Design review of the part built by this model. Coordinates are the model's own, in mm. A direction names the side the tool comes from. Coordinates: 2 decimals unless noted, no trailing zeros. Order: outer loops, then holes, each group sorted by start corner. A loop starts at its lowest first (then second) coordinate and runs counter-clockwise, first axis right, second up. Notation, with made-up numbers: M 89.5,-22.75 L 122.5,-22.75 A18 ccw 122.5,7.25 Z; hole C 66.25,28 d10. An arc over 180 degrees is marked long. Answer as a JSON object with one key per item and string values.
from build123d import *

# Parameters (mm, degrees)
SKETCH1_W           = 60
SKETCH1_H           = 38
BOSS_EXTRUDE1_DEPTH = 35
SKETCH2_R           = 2.9
SKETCH2_R_2         = 3.05
CUT_EXTRUDE1_DEPTH  = 36
SKETCH3_R           = 5.5
CUT_EXTRUDE2_DEPTH  = 7
CHAMFER1_SIZE       = 0.4


with BuildPart() as part:
    # Sketch1 → Boss-Extrude1 (new body)
    with BuildSketch(Plane(origin=(0, 0, 0), x_dir=(1, 0, 0), z_dir=(0, 1, 0))):
        Rectangle(SKETCH1_W, SKETCH1_H)
    extrude(amount=BOSS_EXTRUDE1_DEPTH)

    # Sketch2 → Cut-Extrude1 (cut, through all)
    with BuildSketch(Plane(origin=(0, 35, 0), x_dir=(1, 0, 0), z_dir=(0, 1, 0))):
        with Locations((-23, -9)):
            Circle(SKETCH2_R)
        with Locations((23, -9)):
            Circle(SKETCH2_R)
        with Locations((-15, 11.5)):
            Circle(SKETCH2_R_2)
        with Locations((0, -11.5)):
            Circle(SKETCH2_R_2)
        with Locations((15, 11.5)):
            Circle(SKETCH2_R_2)
    extrude(amount=-CUT_EXTRUDE1_DEPTH, mode=Mode.SUBTRACT)

    # Sketch3 → Cut-Extrude2 (cut)
    with BuildSketch(Plane(origin=(0, 35, 0), x_dir=(1, 0, 0), z_dir=(0, 1, 0))):
        with Locations((-15, 11.5)):
            Circle(SKETCH3_R)
        with Locations((15, 11.5)):
            Circle(SKETCH3_R)
        with Locations((0, -11.5)):
            Circle(SKETCH3_R)
    extrude(amount=-CUT_EXTRUDE2_DEPTH, mode=Mode.SUBTRACT)

    # Chamfer1
    chamfer1_edges = [part.edges().sort_by_distance(p)[0] for p in [
        (30, 35, 0),
        (0, 35, -19),
        (-25.9, 35, 9),
        (20.1, 35, 9),
        (-20.5, 35, -11.5),
        (9.5, 35, -11.5),
        (-5.5, 35, 11.5),
        (-30, 35, 0),
        (0, 0, -19),
        (30, 0, 0),
        (0, 0, 19),
        (-30, 0, 0),
        (-30, 17.5, -19),
        (30, 17.5, -19),
        (30, 17.5, 19),
        (-30, 17.5, 19),
        (0, 35, 19),
    ]]
    chamfer(chamfer1_edges, length=CHAMFER1_SIZE)


solid = part.part
1) Tool access review of faces 1 (the cylindrical face through (-25.9, 17.5, 8.9)), 2 (the cylindrical face through (-16.19, 31.35, -6.13)): name each direction out of +Z, -Z, +X, -X, +Y, -Y from which nothing blocks a thin tool from reaching the whole face with its end or side.
Taken from the geometry:
{"face 1": "+Y, -Y", "face 2": "+Y"}
2) Add section C-C (y = 22). State the section outline as (x, z) points.
Taken from the geometry:
{"outline": "M -30,-18.6 L -29.6,-19 L 29.6,-19 L 30,-18.6 L 30,18.6 L 29.6,19 L -29.6,19 L -30,18.6 Z; hole C -23,9 d5.8; hole C -15,-11.5 d6.1; hole C 0,11.5 d6.1; hole C 15,-11.5 d6.1; hole C 23,9 d5.8"}
3) Add section D-D (x = 15). State the section outline as (y, z) points, and give its area (3 significant figures).
Taken from the geometry:
{"outline": "M 0,-18.6 L 0.4,-19 L 34.6,-19 L 35,-18.6 L 35,-17.4 L 34.6,-17 L 28,-17 L 28,-14.55 L 0,-14.55 Z; M 0,-8.45 L 28,-8.45 L 28,-6 L 34.6,-6 L 35,-5.6 L 35,18.6 L 34.6,19 L 0.4,19 L 0,18.6 Z", "area": "1,080 mm2"}
4) Mouldability with a two-part tool opening along Z and no side actions: class faces 3 (the flat face through (-30, 17, 0)), 4 (the flat face through (0, 17, -19)), 5 (the cylindrical face through (1.64, 14.2, 8.93)), 6 (the flat face through (2, 28, 14)) as released by +Z, released by -Z, zero draft, split by the parting line, or undercut.
Taken from the geometry:
{"face 3": "zero draft", "face 4": "released by -Z", "face 5": "undercut", "face 6": "undercut"}
5) Add section A-A (x = -23). State the section outline as (y, z) points.
Taken from the geometry:
{"outline": "M 0,-18.6 L 0.4,-19 L 34.6,-19 L 35,-18.6 L 35,5.7 L 34.6,6.1 L 0,6.1 Z; M 0,11.9 L 34.6,11.9 L 35,12.3 L 35,18.6 L 34.6,19 L 0.4,19 L 0,18.6 Z"}
6) Insertion check: pin 1 Ø6.5 at (x, z) = (15, -11.5) entering from +Y; pin 2 Ø9.5 at (x, z) = (23, 9) entering from +Y. Each pin has a flat end and moves straight along its axis. Give the tip position at first contact, or say it passes through.
Taken from the geometry:
{"pin 1": "stops at y = 28", "pin 2": "stops at y = 35"}
7) To check wall thickness, follow L1, parallel to X at y = 29.5, z = -11.5; L2, parallel to X at y = 9, z = -11.5; L3, parallel to Z at x = 15, y = 31. State the ranges of each line that lie inside material, in increasing order.
Taken from the geometry:
{"L1": "x = -30 to -20.5, -9.5 to 9.5, 20.5 to 30", "L2": "x = -30 to -18.05, -11.95 to 11.95, 18.05 to 30", "L3": "z = -19 to -17, -6 to 19"}
8) Add section B-B (z = -11.5). State the section outline as (x, y) points, and give its area (3 significant figures).
Taken from the geometry:
{"outline": "M -30,0.4 L -29.6,0 L -18.05,0 L -18.05,28 L -20.5,28 L -20.5,34.6 L -20.9,35 L -29.6,35 L -30,34.6 Z; M -11.95,0 L 11.95,0 L 11.95,28 L 9.5,28 L 9.5,34.6 L 9.1,35 L -9.1,35 L -9.5,34.6 L -9.5,28 L -11.95,28 Z; M 18.05,0 L 29.6,0 L 30,0.4 L 30,34.6 L 29.6,35 L 20.9,35 L 20.5,34.6 L 20.5,28 L 18.05,28 Z", "area": "1,600 mm2"}
